Part model, mm, in its own coordinate system. A direction names the side the tool comes from. Round coordinates to 2 decimals unless told otherwise and drop trailing zeros. Loops run counter-clockwise (first coordinate to the right, second up) from the corner with the lowest first, then second, coordinate; pieces in that order, holes last. Notation, with made-up numbers: (7, 49) -> (21, 49) arc R31 ccw to (21, 73) -> close; hole circle Ø10 at (85.25, 27). An arc over 180 degrees is marked (long way). Use a Markdown table: item, result. Add a question column.
Item 1: Two-plate mould, pull along Z, no slides. Class faces 4 (the face through (7.97, -1.14, -1.94)), 5 (the face through (8, 2.25, 0)), 6 (the face through (8, 0, 0)): pulls with the +Z half, pulls with the -Z half, needs draft (parallel to the pull), parting line crosses it, or undercut.
Item 2: Cut at A-A, the plane z = 0. List the corners of the cut face in (x, y), plus the area to 3 significant figures.
Item 3: Flat gauge pin, fed straight in: pin 1 (1 mm diameter, centred on y = -1, z = -2, fed in from -X). Where does the tip first touch, or does it go through?
Item 4: Cut at D-D, the plane x = 3.25. List the corners of the cut face in (y, z).
Item 5: Probe line 1 (Y direction, x = 9.25, z = 0); line 2 (X direction, y = -0.2, z = 1); line 3 (X direction, y = 1.8, z = -0.65). List the from-to ranges inside material, lowest first. Write a range as [from, to].
Item 6: Cut at B-B, the plane x = 6.5. List the corners of the cut face in (y, z).
Item 7: Cut at C-C, the plane y = -1.05. List the corners of the cut face in (x, z).
Item 8: Which spindle directions (+Z, -Z, +X, -X, +Y, -Y) get a long thin tool onto all of the face, cutting with end or side? Do faces 1 (the face through (7.972, -1.109, 1.958)), 2 (the face through (6, 2, 0)), 3 (the face through (8.99, 0.07, 1.5)). Say none if no direction does.
```python
from build123d import *

# Parameters (mm, degrees)
SKETCH_1_R          = 1.5
EXTRUDE_1_DEPTH     = 6
EXTRUDE_2_DEPTH     = 4
CUT_EXTRUDE_START   = -2
SKETCH_4_R          = 1.5
CUT_EXTRUDE_1_DEPTH = 2


with BuildPart() as part:
    # 草图1 → 凸台-拉伸1 (new body)
    with BuildSketch(Plane(origin=(0, 0, 0), x_dir=(0, 0, -1), z_dir=(1, 0, 0))):
        Circle(SKETCH_1_R)
    extrude(amount=EXTRUDE_1_DEPTH)

    # 草图2 → 凸台-拉伸2 (add)
    with BuildSketch(Plane(origin=(6, 0, 0), x_dir=(0, 0, -1), z_dir=(1, 0, 0))):
        Polygon((2.598076211, 0), (1.299038106, 2.25), (-1.299038106, 2.25), (-2.598076211, 0), (-1.299038106, -2.25), (1.299038106, -2.25), align=None)
    extrude(amount=EXTRUDE_2_DEPTH)

    # 草图4 → 切除-拉伸1 (cut)
    with BuildSketch(Plane(origin=(10, 0, 0), x_dir=(0, 0, -1), z_dir=(1, 0, 0)).offset(CUT_EXTRUDE_START)):
        Circle(SKETCH_4_R)
    extrude(amount=CUT_EXTRUDE_1_DEPTH, mode=Mode.SUBTRACT)


solid = part.part
```
A:
| question | item | result |
|---|---|---|
| 1 | face 4 | pulls with the -Z half |
| 1 | face 5 | needs draft |
| 1 | face 6 | undercut |
| 2 | outline | (0, -1.5) -> (6, -1.5) -> (6, -2.25) -> (10, -2.25) -> (10, -1.5) -> (8, -1.5) -> (8, 1.5) -> (10, 1.5) -> (10, 2.25) -> (6, 2.25) -> (6, 1.5) -> (0, 1.5) -> close |
| 2 | area | 30.0 mm^2 |
| 3 | pin 1 | stops at x = 6 |
| 4 | outline | circle Ø3 at (0, 0) |
| 5 | line 1 | y = [-2.25, -1.5], [1.5, 2.25] |
| 5 | line 2 | x = [0, 8] |
| 5 | line 3 | x = [6, 10] |
| 6 | outline | (-2.25, -1.3) -> (0, -2.6) -> (2.25, -1.3) -> (2.25, 1.3) -> (0, 2.6) -> (-2.25, 1.3) -> close |
| 7 | outline | (0, -1.07) -> (6, -1.07) -> (6, -1.99) -> (10, -1.99) -> (10, -1.07) -> (8, -1.07) -> (8, 1.07) -> (10, 1.07) -> (10, 1.99) -> (6, 1.99) -> (6, 1.07) -> (0, 1.07) -> close |
| 8 | face 1 | +Z, +X, -X, -Y |
| 8 | face 2 | -X |
| 8 | face 3 | +X |
